Check sheet for the modelled part. Datum: model origin and axes. Units: mm. A direction names the side the tool comes from. Round coordinates to 2 decimals unless told otherwise and drop trailing zeros. Loops run counter-clockwise (first coordinate to the right, second up) from the corner with the lowest first, then second, coordinate; pieces in that order, holes last. Notation, with made-up numbers: (64, 31) - (101, 31) arc R10 cw to (101, 49) - close; hole circle Ø5 at (86.25, 20). An arc over 180 degrees is marked (long way). Put each result on its own line as item: value.
```python
from build123d import *

# Parameters (mm, degrees)
CROQUIS1_R              = 13
SALIENTE_EXTRUIR1_DEPTH = 120
CORTAR_EXTRUIR1_DEPTH   = 117.5
REDONDEO1_R             = 20
CROQUIS3_W              = 250
CROQUIS3_H              = 250
CORTAR_EXTRUIR2_DEPTH   = 312.295872079
CORTAR_EXTRUIR4_DEPTH   = 5
CROQUIS7_R              = 2.75
CROQUIS7_R_2            = 2
CORTAR_EXTRUIR5_DEPTH   = 6
REDONDEO5_R             = 10
CROQUIS8_W              = 4
CROQUIS8_H              = 30
CORTAR_EXTRUIR6_DEPTH   = 15
REDONDEO6_R             = 2
CROQUIS9_R              = 2.25
SALIENTE_EXTRUIR3_DEPTH = 6
CROQUIS10_R             = 1.5
SALIENTE_EXTRUIR4_DEPTH = 3
CROQUIS11_R             = 2
SALIENTE_EXTRUIR5_DEPTH = 3


with BuildPart() as part:
    # Croquis1 → Saliente-Extruir1 (new body)
    with BuildSketch(Plane(origin=(0, 0, 0), x_dir=(0, 0, -1), z_dir=(1, 0, 0))):
        with BuildLine():
            Line((-210, 0), (210, 0))
            Line((210, 0), (210, 45))
            Line((210, 45), (185, 70))
            Line((185, 70), (21.52779525, 70))
            Line((21.52779525, 70), (21.52779525, 75))
            Line((21.52779525, 75), (-28.77527986, 148.293505427))
            ThreePointArc((-28.77527986, 148.293505427), (-68.645544514, 169.981651137), (-109.631887894, 150.484643051))
            Line((-109.631887894, 150.484643051), (-210, 20))
            Line((-210, 20), (-210, 0))
        make_face()
        with Locations((-70, 120)):
            Circle(CROQUIS1_R, mode=Mode.SUBTRACT)
    extrude(amount=-SALIENTE_EXTRUIR1_DEPTH)

    # Croquis2 → Cortar-Extruir1 (cut)
    with BuildSketch(Plane.ZY.offset(120)):
        with BuildLine():
            Line((106.461336862, 148.045871607), (206, 18.639562604))
            Line((206, 18.639562604), (206, 0))
            Line((206, 0), (-206, 0))
            Line((-206, 0), (-206, 43.343145751))
            Line((-206, 43.343145751), (-183.343145751, 66))
            Line((-183.343145751, 66), (-37.52779525, 66))
            Line((-37.52779525, 66), (-37.52779525, 60))
            Line((-37.52779525, 60), (-17.52779525, 60))
            Line((-17.52779525, 60), (-17.52779525, 73.759393051))
            Line((-17.52779525, 73.759393051), (32.073257471, 146.030024993))
            ThreePointArc((32.073257471, 146.030024993), (68.753900953, 165.983119046), (106.461336862, 148.045871607))
        make_face()
    extrude(amount=-CORTAR_EXTRUIR1_DEPTH, mode=Mode.SUBTRACT)

    # Redondeo1
    redondeo1_edges = [part.edges().sort_by_distance(p)[0] for p in [
        (-60, 20, 210),
        (-60, 70, -185),
        (-60, 45, -210),
        (-61.25, 66, -183.343145751),
        (-61.25, 43.343145751, -206),
        (-61.25, 18.639562604, 206),
    ]]
    fillet(redondeo1_edges, radius=REDONDEO1_R)

    # Croquis3 → Cortar-Extruir2 (cut, through all)
    with BuildSketch(Plane(origin=(0, 0, -21.52779525), x_dir=(-1, 0, 0), z_dir=(0, 0, -1))):
        with Locations((60, 70)):
            Rectangle(CROQUIS3_W, CROQUIS3_H)
    extrude(amount=-CORTAR_EXTRUIR2_DEPTH, mode=Mode.SUBTRACT)

    # Croquis6 → Cortar-Extruir4 (cut)
    with BuildSketch(Plane.ZY.offset(120)):
        with BuildLine():
            Line((-23.02779525, 61.5), (-23.02779525, 68.5))
            Line((-23.02779525, 68.5), (-176.715728753, 68.5))
            ThreePointArc((-176.715728753, 68.5), (-183.795372251, 67.091771351), (-189.797204204, 63.081475452))
            Line((-189.797204204, 63.081475452), (-203.081475452, 49.797204204))
            ThreePointArc((-203.081475452, 49.797204204), (-207.091771351, 43.795372251), (-208.5, 36.715728753))
            Line((-208.5, 36.715728753), (-208.5, 1.5))
            Line((-208.5, 1.5), (-207.5, 1.5))
            Line((-207.5, 1.5), (-207.5, 35.058874503))
            ThreePointArc((-207.5, 35.058874503), (-205.863409949, 43.286568299), (-201.202795796, 50.261670299))
            Line((-201.202795796, 50.261670299), (-190.261670299, 61.202795796))
            ThreePointArc((-190.261670299, 61.202795796), (-183.286568299, 65.863409949), (-175.058874503, 67.5))
            Line((-175.058874503, 67.5), (-36.02779525, 67.5))
            Line((-36.02779525, 67.5), (-36.02779525, 61.5))
            Line((-36.02779525, 61.5), (-23.02779525, 61.5))
        make_face()
    extrude(amount=-CORTAR_EXTRUIR4_DEPTH, mode=Mode.SUBTRACT)

    # Croquis7 → Cortar-Extruir5 (cut)
    with BuildSketch(Plane.XY.offset(-21.52779525)):
        with Locations((-40, 64)):
            Circle(CROQUIS7_R)
        with Locations((-100, 64)):
            Circle(CROQUIS7_R)
        with Locations((-70, 64)):
            Circle(CROQUIS7_R_2)
        with Locations((-10, 64)):
            Circle(CROQUIS7_R_2)
    extrude(amount=-CORTAR_EXTRUIR5_DEPTH, mode=Mode.SUBTRACT)

    # Redondeo5
    redondeo5_edges = [part.edges().sort_by_distance(p)[0] for p in [
        (0, 18.357864376, -210),
        (0, 44.3693974, -208.47759065),
        (0, 57.5, -197.5),
        (0, 68.47759065, -184.3693974),
        (0, 70, -99.121762001),
        (-2.5, 17.529437252, -206),
        (-2.5, 42.71254315, -204.47759065),
        (-2.5, 54.671572875, -194.671572875),
        (-2.5, 64.47759065, -182.71254315),
        (-2.5, 66, -106.293334877),
    ]]
    fillet(redondeo5_edges, radius=REDONDEO5_R)

    # Croquis8 → Cortar-Extruir6 (cut)
    with BuildSketch(Plane(origin=(0, 0, -210), x_dir=(-1, 0, 0), z_dir=(0, 0, -1))):
        with Locations((110, 18)):
            Rectangle(CROQUIS8_W, CROQUIS8_H)
        with Locations((100.9, 18)):
            Rectangle(CROQUIS8_W, CROQUIS8_H)
        with Locations((91.8, 18)):
            Rectangle(CROQUIS8_W, CROQUIS8_H)
        with Locations((82.7, 18)):
            Rectangle(CROQUIS8_W, CROQUIS8_H)
        with Locations((73.6, 18)):
            Rectangle(CROQUIS8_W, CROQUIS8_H)
        with Locations((64.5, 18)):
            Rectangle(CROQUIS8_W, CROQUIS8_H)
        with Locations((55.4, 18)):
            Rectangle(CROQUIS8_W, CROQUIS8_H)
        with Locations((46.3, 18)):
            Rectangle(CROQUIS8_W, CROQUIS8_H)
        with Locations((37.2, 18)):
            Rectangle(CROQUIS8_W, CROQUIS8_H)
        with Locations((28.1, 18)):
            Rectangle(CROQUIS8_W, CROQUIS8_H)
        with Locations((19, 18)):
            Rectangle(CROQUIS8_W, CROQUIS8_H)
    extrude(amount=-CORTAR_EXTRUIR6_DEPTH, mode=Mode.SUBTRACT)

    # Redondeo6
    redondeo6_edges = [part.edges().sort_by_distance(p)[0] for p in [
        (-21, 3, -208),
        (-17, 3, -208),
        (-17, 33, -208),
        (-30.1, 3, -208),
        (-26.1, 3, -208),
        (-26.1, 33, -208),
        (-30.1, 33, -208),
        (-39.2, 3, -208),
        (-35.2, 3, -208),
        (-35.2, 33, -208),
        (-39.2, 33, -208),
        (-48.3, 3, -208),
        (-44.3, 3, -208),
        (-44.3, 33, -208),
        (-48.3, 33, -208),
        (-57.4, 3, -208),
        (-53.4, 3, -208),
        (-53.4, 33, -208),
        (-57.4, 33, -208),
        (-66.5, 3, -208),
        (-62.5, 3, -208),
        (-62.5, 33, -208),
        (-66.5, 33, -208),
        (-75.6, 3, -208),
        (-71.6, 3, -208),
        (-71.6, 33, -208),
        (-75.6, 33, -208),
        (-84.7, 3, -208),
        (-80.7, 3, -208),
        (-80.7, 33, -208),
        (-84.7, 33, -208),
        (-93.8, 3, -208),
        (-89.8, 3, -208),
        (-89.8, 33, -208),
        (-93.8, 33, -208),
        (-102.9, 3, -208),
        (-98.9, 3, -208),
        (-98.9, 33, -208),
        (-102.9, 33, -208),
        (-112, 33, -208),
        (-112, 3, -208),
        (-108, 3, -208),
        (-108, 33, -208),
        (-21, 33, -208),
    ]]
    fillet(redondeo6_edges, radius=REDONDEO6_R - 0.0001)  # a hair under: the kernel refuses the full size

    # Croquis9 → Saliente-Extruir3 (add)
    with BuildSketch(Plane.XZ):
        with BuildLine():
            Line((-2.5, -125), (-5, -125))
            ThreePointArc((-5, -125), (-10, -130), (-5, -135))
            Line((-5, -135), (-2.5, -135))
            Line((-2.5, -135), (-2.5, -125))
        make_face()
        with Locations(Location((-5, -130, 0), (0, 0, 270))):
            Circle(CROQUIS9_R, mode=Mode.SUBTRACT)
    extrude(amount=-SALIENTE_EXTRUIR3_DEPTH)

    # Croquis10 → Saliente-Extruir4 (add)
    with BuildSketch(Plane.ZY.offset(120)):
        with BuildLine():
            Line((-210, 0), (-216, 0))
            ThreePointArc((-216, 0), (-221, 5), (-216, 10))
            Line((-216, 10), (-210, 10))
            Line((-210, 10), (-210, 0))
        make_face()
        with Locations((-216, 5)):
            Circle(CROQUIS10_R, mode=Mode.SUBTRACT)
    extrude(amount=-SALIENTE_EXTRUIR4_DEPTH)

    # Croquis11 → Saliente-Extruir5 (add)
    with BuildSketch(Plane.XY.offset(-21.52779525)):
        with BuildLine():
            Line((-2.5, 15), (-7, 15))
            ThreePointArc((-7, 15), (-12, 20), (-7, 25))
            Line((-7, 25), (-2.5, 25))
            Line((-2.5, 25), (-2.5, 15))
        make_face()
        with Locations((-7, 20)):
            Circle(CROQUIS11_R, mode=Mode.SUBTRACT)
    extrude(amount=-SALIENTE_EXTRUIR5_DEPTH)


solid = part.part
```
Item 1: Section check B-B on y = 20. Count the separate pieces of the cut face and the enclosed holes in it, then the cut area to 3 significant figures.
Filled sheet:
separate pieces: 13
enclosed holes: 0
area: 777 mm²
Item 2: Thickness scan on line 1 (Y direction, x = -7, z = -23.3); line 2 (Y direction, x = -66, z = -59); line 3 (X direction, y = 31.5, z = -86.5). Record the ranges inside material, lowest first. Write a range as from..to.
Filled sheet:
line 1: 15..18, 22..25, 60..69.54
line 2: 66..70
line 3: -2.5..0
Item 3: Release check for a two-part mould opening along X. For faces 1 (the flat face through (-62.5, 18, -208)), 2 (the flat face through (0, 30, -110)), 3 (the flat face through (-84.7, 18, -208)), 4 (the cylindrical face through (-65.77, 44.27, -208.52)) record: +X half, -X half, draft (parallel to the pull), parting line (faces both ways), or undercut.
Filled sheet:
face 1: undercut
face 2: +X half
face 3: undercut
face 4: draft
Item 4: Go/stop test with flat-tipped pins: pin 1 (1.5 mm diameter, centred on x = -5, z = -23.5, fed in from -Y); pin 2 (5 mm diameter, centred on x = -89, y = 41.5, fed in from -Z); pin 3 (2 mm diameter, centred on x = -9.5, y = 63.5, fed in from +Z). Record where each tip stops, or that it passes through.
Filled sheet:
pin 1: y = 15
pin 2: z = -209.87
pin 3: z = -27.53
Item 5: Section check A-A on z = -165. Enter the section's corners in (x, y).
Filled sheet:
outline: (-120, 66) - (-12.5, 66) arc R10 cw to (-2.5, 56) - (-2.5, 0) - (0, 0) - (0, 60) arc R10 ccw to (-10, 70) - (-120, 70) - (-120, 68.5) - (-115, 68.5) - (-115, 67.5) - (-120, 67.5) - close
Item 6: Tool access check on faces 5 (the flat face through (-118, 19, -208.5)), 6 (the flat face through (-120, 66.3, -135.6)), 7 (the flat face through (-64, 57, -198)), 8 (the flat face through (-80.7, 18, -208)), 9 (the cylindrical face through (-100.358, 66.727, -24.486)). Record the directions out of +Z, -Z, +X, -X, +Y, -Y that give a thin tool (end or side, any length) a straight path to the whole face; none if there is none.
Filled sheet:
face 5: -X
face 6: +Z, -Z, -X, +Y, -Y
face 7: -Z, +X, -X, +Y
face 8: +Z, -Z
face 9: +Z
